Part model, mm, in its own coordinate system. Give positions to 0.01 mm unless a question says otherwise; leave off trailing zeros. Order: outer loops, then holes, each group sorted by start corner. A loop starts at its lowest first (then second) coordinate and runs counter-clockwise, first axis right, second up. Notation, with made-up numbers: (49, 48) - (95, 48) arc R36 ccw to (95, 85) - close; hole circle Ø3 at (-39, 35.5). An arc over 180 degrees is marked (long way). One line per item, written item: value.
Autodesk Inventor part; units mm, degrees
ref_plane "black_body_str_XY" through (0, 8.8392, 0) normal (0, -1, 0) x (1, 0, 0)
ref_plane "black_body_str_YZ" through (0, 8.8392, 0) normal (1, 0, 0) x (0, 0, 1)
ref_plane "black_body_str_ZX" through (0, 8.8392, 0) normal (0, 0, 1) x (0, -1, 0)
sketch "Sketch_1" plane through (0, 0, 0) normal (0, 1, 0) x (-1, 0, 0)
  line L0 (3.4036, -4.1402) -> (3.4036, 4.1402)
  arc A0 (3.4036, 4.1402) -> (3.1496, 4.3942) centre (3.1496, 4.1402) ccw
  line L1 (3.1496, 4.3942) -> (-3.1496, 4.3942)
  arc A1 (-3.1496, 4.3942) -> (-3.4036, 4.1402) centre (-3.1496, 4.1402) ccw
  line L2 (-3.4036, 4.1402) -> (-3.4036, -4.1402)
  arc A2 (-3.4036, -4.1402) -> (-3.1496, -4.3942) centre (-3.1496, -4.1402) ccw
  line L3 (-3.1496, -4.3942) -> (3.1496, -4.3942)
  arc A3 (3.1496, -4.3942) -> (3.4036, -4.1402) centre (3.1496, -4.1402) ccw
extrude "Extrusion1" add sketch "Sketch_1" along normal blind 8.8392
sketch "Sketch_2" plane through (0, 8.8392, 0) normal (0, 1, 0) x (1, 0, 0)
  line L0 (-7.3539, 7.1515) -> (-7.3539, -8.5008)
  line L1 (-7.3539, -8.5008) -> (8.5233, -8.5008)
  line L2 (8.5233, -8.5008) -> (8.5233, 7.1515)
  line L3 (8.5233, 7.1515) -> (-7.3539, 7.1515)
  line L4 (-2.9972, -3.9878) -> (2.9972, -3.9878)
  line L5 (2.9972, -3.9878) -> (2.9972, 3.9878)
  line L6 (2.9972, 3.9878) -> (-2.9972, 3.9878)
  line L7 (-2.9972, 3.9878) -> (-2.9972, -3.9878)
extrude "Extrusion2" cut sketch "Sketch_2" against normal blind 3.6576
sketch "Sketch_3" plane through (3.4036, 0, 0) normal (1, 0, 0) x (0, 0, -1)
  line L0 (-3.6068, 0) -> (3.6068, 0)
  line L1 (3.6068, 0) -> (3.6068, 0.7874)
  line L2 (3.6068, 0.7874) -> (-3.6068, 0.7874)
  line L3 (-3.6068, 0.7874) -> (-3.6068, 0)
extrude "Extrusion3" cut sketch "Sketch_3" against normal blind 6.8072
sketch "Sketch_4" plane through (0, 0, 4.3942) normal (0, 0, 1) x (1, 0, 0)
  line L0 (-2.6162, 0) -> (2.6162, 0)
  line L1 (2.6162, 0) -> (2.6162, 0.7874)
  line L2 (2.6162, 0.7874) -> (-2.6162, 0.7874)
  line L3 (-2.6162, 0.7874) -> (-2.6162, 0)
extrude "Extrusion4" cut sketch "Sketch_4" against normal blind 8.7884
sketch "Sketch_5" plane through (3.4036, 0, 0) normal (1, 0, 0) x (0, 0, -1)
  line L0 (-3.3782, 5.1816) -> (-3.3782, 3.9116)
  line L1 (-3.3782, 3.9116) -> (3.3782, 3.9116)
  line L2 (3.3782, 3.9116) -> (3.3782, 5.1816)
  line L3 (3.3782, 5.1816) -> (-3.3782, 5.1816)
extrude "Extrusion5" cut sketch "Sketch_5" against normal blind 0.4064
sketch "Sketch_6" plane through (-3.4036, 0, 0) normal (1, 0, 0) x (0, 0, -1)
  line L0 (-3.3782, 5.1816) -> (-3.3782, 3.9116)
  line L1 (-3.3782, 3.9116) -> (3.3782, 3.9116)
  line L2 (3.3782, 3.9116) -> (3.3782, 5.1816)
  line L3 (3.3782, 5.1816) -> (-3.3782, 5.1816)
extrude "Extrusion6" cut sketch "Sketch_6" along normal blind 0.4064
sketch "Sketch_7" plane through (0, 0, 4.3942) normal (0, 0, 1) x (1, 0, 0)
  line L0 (-2.3622, 5.1816) -> (-2.3622, 3.9116)
  line L1 (-2.3622, 3.9116) -> (2.3622, 3.9116)
  line L2 (2.3622, 3.9116) -> (2.3622, 5.1816)
  line L3 (2.3622, 5.1816) -> (-2.3622, 5.1816)
extrude "Extrusion7" cut sketch "Sketch_7" against normal blind 0.4064
sketch "Sketch_8" plane through (0, 0, -4.3942) normal (0, 0, 1) x (1, 0, 0)
  line L0 (-2.3622, 5.1816) -> (-2.3622, 3.9116)
  line L1 (-2.3622, 3.9116) -> (2.3622, 3.9116)
  line L2 (2.3622, 3.9116) -> (2.3622, 5.1816)
  line L3 (2.3622, 5.1816) -> (-2.3622, 5.1816)
extrude "Extrusion8" cut sketch "Sketch_8" along normal blind 0.4064
sketch "Sketch_49" plane through (0, 0.7874, 0) normal (0, 1, 0) x (1, 0, 0)
  line L0 (-2.6162, -3.6068) -> (2.6162, -3.6068)
  line L1 (2.6162, -3.6068) -> (2.6162, 3.6068)
  line L2 (2.6162, 3.6068) -> (-2.6162, 3.6068)
  line L3 (-2.6162, 3.6068) -> (-2.6162, -3.6068)
extrude "Extrusion9" cut sketch "Sketch_49" along normal blind 0.0254
ref_plane "black_body_str_XY" through (0, 8.8392, 0) normal (0, -1, 0) x (1, 0, 0)
ref_plane "black_body_str_YZ" through (0, 8.8392, 0) normal (1, 0, 0) x (0, 0, 1)
ref_plane "black_body_str_ZX" through (0, 8.8392, 0) normal (0, 0, 1) x (0, -1, 0)
ref_plane "black_body_ver_rigang_XY" through (0, 0, 9.0678) normal (0, 0, -1) x (1, 0, 0)
ref_plane "black_body_ver_rigang_YZ" through (0, 0, 9.0678) normal (1, 0, 0) x (0, -1, 0)
ref_plane "black_body_ver_rigang_ZX" through (0, 0, 9.0678) normal (0, -1, 0) x (0, 0, -1)
ref_plane "dummy_righ_vert_XY" through (0, 0, 0) normal (0, 0, -1) x (1, 0, 0)
ref_plane "dummy_righ_vert_YZ" through (0, 0, 0) normal (1, 0, 0) x (0, -1, 0)
ref_plane "dummy_righ_vert_ZX" through (0, 0, 0) normal (0, -1, 0) x (0, 0, -1)
ref_plane "dummy_straight_XY" through (0, 0, 0) normal (0, -1, 0) x (1, 0, 0)
ref_plane "dummy_straight_YZ" through (0, 0, 0) normal (1, 0, 0) x (0, 0, 1)
ref_plane "dummy_straight_ZX" through (0, 0, 0) normal (0, 0, 1) x (0, -1, 0)
ref_plane "rigang_vert_trmnls_XY" through (0, 0, 0.8636) normal (0, 0, 1) x (1, 0, 0)
ref_plane "rigang_vert_trmnls_YZ" through (0, 0, 0.8636) normal (1, 0, 0) x (0, 1, 0)
ref_plane "rigang_vert_trmnls_ZX" through (0, 0, 0.8636) normal (0, 1, 0) x (0, 0, 1)
ref_plane "str_trmnls_XY" through (0, 0.8636, 0) normal (0, 1, 0) x (1, 0, 0)
ref_plane "str_trmnls_YZ" through (0, 0.8636, 0) normal (1, 0, 0) x (0, 0, -1)
ref_plane "str_trmnls_ZX" through (0, 0.8636, 0) normal (0, 0, -1) x (0, 1, 0)
properties part number "B12APbody"
1) Drop a flat-ended pin along its axis: P1, Ø0.6, axis at x = -3, z = -1.5, coming from the -Y side. Give the stop position or say it passes through.
Answer:
P1: stops at y = 0.79
2) Two-plate mould, pull along X, no slides. Class faces 1 (the face through (3.404, 3, 0)), 2 (the face through (0, 0.813, 0)), 3 (the face through (-3.404, 3, 0)), 4 (the face through (0, 3, -4.394)): pulls with the +X half, pulls with the -X half, needs draft (parallel to the pull), parting line crosses it, or undercut.
Answer:
face 1: pulls with the +X half
face 2: undercut
face 3: pulls with the -X half
face 4: needs draft
3) Slice it at C-C on y = 5.75. Write the cut outline in (x, z), then the cut area to 3 significant figures.
Answer:
outline: (-3, -3.99) - (3, -3.99) - (3, 3.99) - (-3, 3.99) - close
area: 47.8 mm2
4) Wall check: line 1 along X through (y, z) = (0.5, -3.75); line 2 along Y through (x, z) = (-1, 2.5); line 3 along X through (y, z) = (4.75, 0.25). Give the ranges that are in metal, low to high. Write a range as [from, to].
Answer:
line 1: x = [-3.4, -2.62], [2.62, 3.4]
line 2: y = [0.81, 8.84]
line 3: x = [-3, 3]
